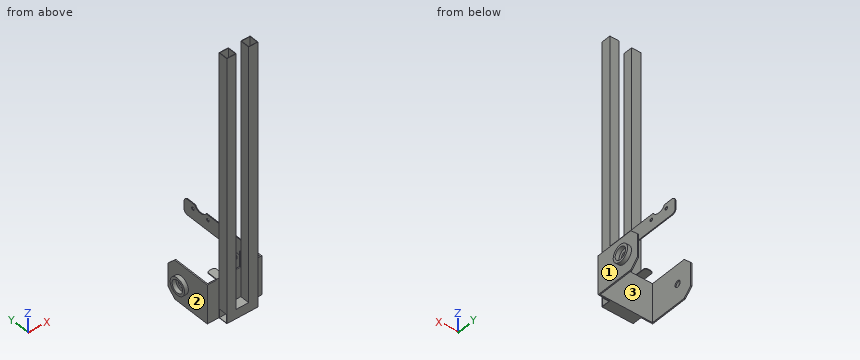
```python
from build123d import *

# Parameters (mm, degrees)
BOSS_EXTRUDE1_DEPTH      = 50
CHAMFER1_SIZE            = 10
SKETCH2_R                = 4
CUT_EXTRUDE1_DEPTH       = 80
SKETCH3_R                = 11
SKETCH3_R_2              = 8
BOSS_EXTRUDE2_DEPTH      = 5
SKETCH4_W                = 12
SKETCH4_H                = 12
SKETCH4_W_2              = 11
SKETCH4_H_2              = 11
BOSS_EXTRUDE3_DEPTH      = 340
SKETCH5_W                = 40
SKETCH5_H                = 12
BOSS_EXTRUDE4_DEPTH      = 12
SKETCH6_W                = 11
SKETCH6_H                = 11
CUT_EXTRUDE2_DEPTH       = 67
BOSS_EXTRUDE5_DEPTH      = 20
FILLET1_R                = 5
SKETCH8_R                = 2
CUT_EXTRUDE3_DEPTH       = 20
BOSS_EXTRUDE6_DEPTH      = 3
BOSS_EXTRUDE6_DEPTH_BACK = 7
SKETCH9_W                = 1
SKETCH9_H                = 15
FILLET2_R                = 3


with BuildPart() as part:
    # Sketch1 → Boss-Extrude1 (new body)
    with BuildSketch(Plane.XY):
        Polygon((-65.816488176, 13.044356197), (-65.816488176, -46.955643803), (4.183511824, -46.955643803), (4.183511824, 13.044356197), (2.683511824, 13.044356197), (2.683511824, -45.455643803), (-64.316488176, -45.455643803), (-64.316488176, 13.044356197), align=None)
    extrude(amount=BOSS_EXTRUDE1_DEPTH)

    # Chamfer1
    chamfer1_edges = [part.edges().sort_by_distance(p)[0] for p in [
        (-65.066488176, 13.044356197, 0),
        (3.433511824, 13.044356197, 50),
        (-65.066488176, 13.044356197, 50),
        (3.433511824, 13.044356197, 0),
    ]]
    chamfer(chamfer1_edges, length=CHAMFER1_SIZE)

    # Sketch2 → Cut-Extrude1 (cut)
    with BuildSketch(Plane(origin=(4.183511824, 0, 0), x_dir=(0, 0, -1), z_dir=(1, 0, 0))):
        with Locations((-25, -6.955643803)):
            Circle(SKETCH2_R)
    extrude(amount=-CUT_EXTRUDE1_DEPTH, mode=Mode.SUBTRACT)

    # Sketch3 → Boss-Extrude2 (add)
    with BuildSketch(Plane(origin=(4.183511824, 0, 0), x_dir=(0, 0, -1), z_dir=(1, 0, 0))):
        with Locations(Location((-25, -6.955643803, 0), (0, 0, 180))):
            Circle(SKETCH3_R)
        with Locations((-25, -6.955643803)):
            Circle(SKETCH3_R_2, mode=Mode.SUBTRACT)
    boss_extrude2 = extrude(amount=BOSS_EXTRUDE2_DEPTH)

    # Mirror1: Boss-Extrude2 across plane
    add(boss_extrude2.mirror(Plane.ZY.offset(30.816488176)))

    # Sketch4 → Boss-Extrude3 (add)
    with BuildSketch(Plane(origin=(0, 0, 0), x_dir=(-1, 0, 0), z_dir=(0, 0, -1))):
        with Locations((16.816488176, -52.955643803)):
            Rectangle(SKETCH4_W, SKETCH4_H)
        with Locations((16.816488176, -52.955643803)):
            Rectangle(SKETCH4_W_2, SKETCH4_H_2, mode=Mode.SUBTRACT)
    boss_extrude3 = extrude(amount=-BOSS_EXTRUDE3_DEPTH)

    # Mirror2: Boss-Extrude3 across plane
    add(boss_extrude3.mirror(Plane.ZY.offset(30.816488176)))

    # Sketch5 → Boss-Extrude4 (add)
    with BuildSketch(Plane(origin=(0, 0, 0), x_dir=(-1, 0, 0), z_dir=(0, 0, -1))):
        with Locations((30.816488176, -52.955643803)):
            Rectangle(SKETCH5_W, SKETCH5_H)
    extrude(amount=-BOSS_EXTRUDE4_DEPTH)

    # Sketch6 → Cut-Extrude2 (cut)
    with BuildSketch(Plane(origin=(-10.816488176, 0, 0), x_dir=(0, 0, -1), z_dir=(1, 0, 0))):
        with Locations((-6, -52.955643803)):
            Rectangle(SKETCH6_W, SKETCH6_H)
    extrude(amount=-CUT_EXTRUDE2_DEPTH, mode=Mode.SUBTRACT)

    # Sketch7 → Boss-Extrude5 (add)
    with BuildSketch(Plane.XY.offset(50)):
        Polygon((-23.570169561, -45.955643803), (-11.816488176, -45.955643803), (-11.816488176, 53.044356197), (-10.816488176, 53.044356197), (-10.816488176, -46.955643803), (-23.570169561, -46.955643803), align=None)
    extrude(amount=BOSS_EXTRUDE5_DEPTH)

    # Fillet1
    fillet1_edges = [part.edges().sort_by_distance(p)[0] for p in [
        (-11.316488176, 53.044356197, 50),
        (-11.316488176, 53.044356197, 70),
    ]]
    fillet(fillet1_edges, radius=FILLET1_R)

    # Sketch8 → Cut-Extrude3 (cut)
    with BuildSketch(Plane(origin=(-10.816488176, 0, 0), x_dir=(0, 0, -1), z_dir=(1, 0, 0))):
        with Locations(Location((-63.5, 39.544356197, 0), (0, 0, 90))):
            Circle(SKETCH8_R)
        with BuildLine():
            Line((-70, 28.044356197), (-70, 19.384102159))
            ThreePointArc((-70, 19.384102159), (-66.339745962, 23.044356197), (-65, 28.044356197))
            ThreePointArc((-65, 28.044356197), (-66.339745962, 33.044356197), (-70, 36.704610234))
            Line((-70, 36.704610234), (-70, 28.044356197))
        make_face()
        with Locations(Location((-63.5, 16.544356197, 0), (0, 0, 90))):
            Circle(SKETCH8_R)
    extrude(amount=-CUT_EXTRUDE3_DEPTH, mode=Mode.SUBTRACT)

    # Sketch9 → Boss-Extrude6 (add, two sides: drawn at the far end of the back side and taken through both)
    with BuildSketch(Plane.ZY.offset(50.816488176).offset(-BOSS_EXTRUDE6_DEPTH_BACK)):
        with Locations((50.5, -39.455643803)):
            Rectangle(SKETCH9_W, SKETCH9_H)
    extrude(amount=BOSS_EXTRUDE6_DEPTH + BOSS_EXTRUDE6_DEPTH_BACK)

    # Fillet2
    fillet2_edges = [part.edges().sort_by_distance(p)[0] for p in [
        (-43.816488176, -31.955643803, 50.5),
        (-53.816488176, -31.955643803, 50.5),
    ]]
    fillet(fillet2_edges, radius=FILLET2_R)


solid = part.part
```
Here's how the part is built. I have some questions about the finished solid (model axes, mm). Face numbers are marked on the shaded views. Give positions to 0.01 mm unless a question says otherwise; leave off trailing zeros. Order: outer loops, then holes, each group sorted by start corner. A loop starts at its lowest first (then second) coordinate and runs counter-clockwise, first axis right, second up. Notation, with made-up numbers: (27, -24.75) -> (36, -24.75) arc R17 ccw to (36, 8.25) -> close; hole circle Ø7 at (16, 33.25). An arc over 180 degrees is marked (long way). Use CSV: the item, a comma, the result in double quotes. Start each with the question number.
Item 1: If I drill on probe 1 along X at (y, z) = (-49, 35.5); probe 2 along Y at (x, z) = (3.95, 25); probe 3 along Y at (x, z) = (-45, 225.5), over which ranges is the centre line in solid material (lowest first)? Write a range as [from, to].
Item 2: Thinking about a two-plate mould opening in X: for the marked faces 1, 2 and 3, which applies, pulls with the +X half, pulls with the -X half, needs draft (parallel to the pull), parting line crosses it, or undercut?
Item 3: Suppose I cut it at A-A (z = 112.5). List the corners of the cut face in (x, y) for me.
Item 4: Suppose I cut it at B-B (x = -15). List the corners of the cut face in (y, z) for me, and give its area (3 significant figures).
Item 5: I'm going to push flat-ended pins straight in: P1, Ø4.5, axis at x = -57, z = 38, coming from the -Y side; P2, Ø3.5, axis at x = -26.5, z = 5.5, coming from the +Y side; P3, Ø5, axis at x = -36.5, z = 135, coming from the -Y side; P4, Ø3.5, axis at x = -47, z = 243.5, coming from the +Y side. Where does each tip first touch, or does it pass through?
Item 6: Suppose I cut it at D-D (y = 23). List the corners of the cut face in (x, z) for me.
Item 7: Suppose I cut it at C-C (z = 25). Give the number of separate pieces and of enclosed holes in the cut face, and give its area (4 significant figures).
Answer block:
1,probe 1,"x = [-50.82, -50.32], [-39.32, -38.82], [-22.82, -22.32], [-11.32, -10.82]"
1,probe 2,"y = [-46.96, -10.96], [-2.96, 13.04]"
1,probe 3,"y = [-58.96, -58.46], [-47.46, -46.96]"
2,face 1,"pulls with the +X half"
2,face 2,"pulls with the -X half"
2,face 3,"undercut"
3,outline,"(-50.82, -58.96) -> (-38.82, -58.96) -> (-38.82, -46.96) -> (-50.82, -46.96) -> close; (-22.82, -58.96) -> (-10.82, -58.96) -> (-10.82, -46.96) -> (-22.82, -46.96) -> close; hole (-50.32, -58.46) -> (-39.32, -58.46) -> (-39.32, -47.46) -> (-50.32, -47.46) -> close; hole (-22.32, -58.46) -> (-11.32, -58.46) -> (-11.32, -47.46) -> (-22.32, -47.46) -> close"
4,outline,"(-58.96, 0) -> (-45.46, 0) -> (-45.46, 50) -> (-45.96, 50) -> (-45.96, 70) -> (-46.96, 70) -> (-46.96, 340) -> (-47.46, 340) -> (-47.46, 12) -> (-58.46, 12) -> (-58.46, 340) -> (-58.96, 340) -> close; hole (-58.46, 0.5) -> (-47.46, 0.5) -> (-47.46, 11.5) -> (-58.46, 11.5) -> close"
4,area,"446 mm^2"
5,P1,"stops at y = -46.96"
5,P2,"stops at y = -45.46"
5,P3,"stops at y = -58.96"
5,P4,"stops at y = -46.96"
6,outline,"(-11.82, 50) -> (-10.82, 50) -> (-10.82, 66.37) -> (-11.82, 66.37) -> close"
7,separate pieces,"3"
7,enclosed holes,"2"
7,area,"362.5 mm^2"
